Source: three-view drawing plus pictorial views. Frame: mm from the lowest corner of the part. Give positions to 0.01 mm unless a question says otherwise; leave off trailing zeros. Loops run counter-clockwise (first coordinate to the right, second up) from the corner with the lowest first, then second, coordinate; pieces in that order, holes last. Notation, with made-up numbers: (-37.75, 88.5) - (10.25, 88.5) arc R17 cw to (10.25, 98.5) - close; hole circle Ø2 at (77, -3). An arc over 180 degrees is marked (long way). Answer in a Markdown table with one row per item.
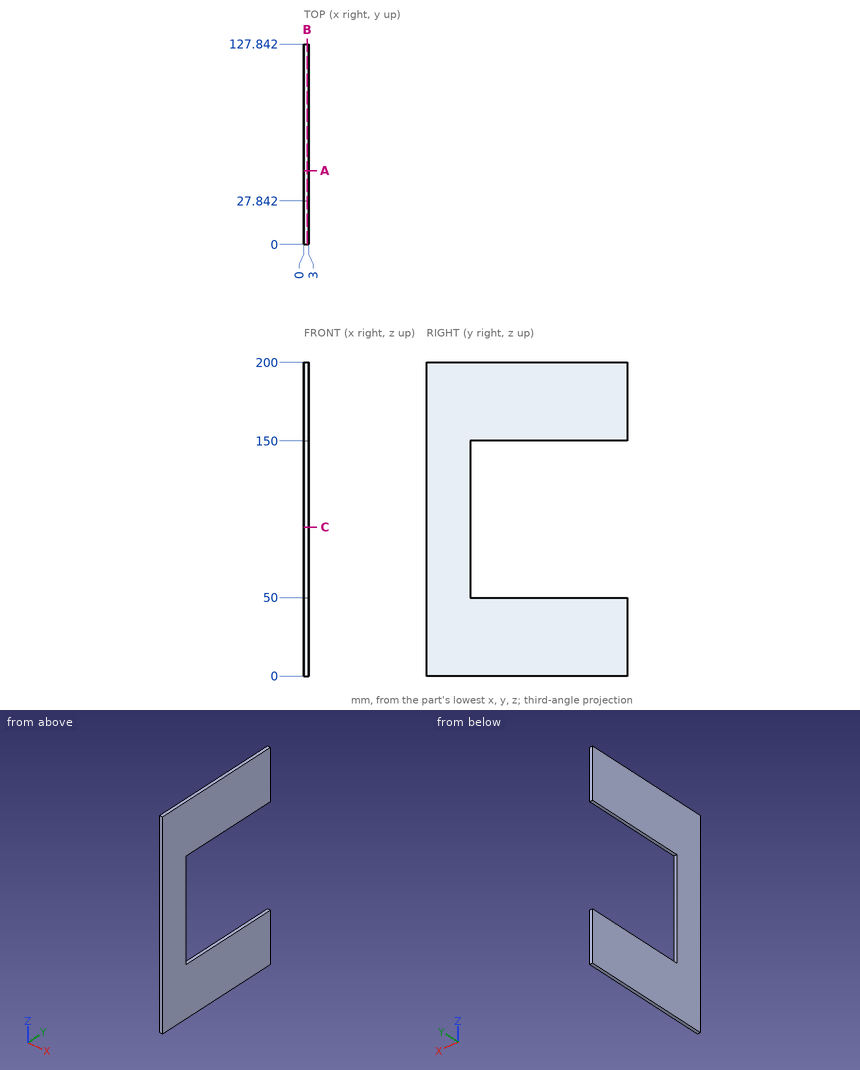
Q1. Material intervals for line 1 along Z through (x, y) = (1.8, 73.5); line 2 along Y through (x, z) = (1.45, 64.5), sorted ascending.
Check values:
| item | result |
|---|---|
| line 1 | 0 to 50, 150 to 200 |
| line 2 | 0 to 27.84 |
Q2. First-contact query: pin 1 (1.5 mm diameter, centred on x = 2, z = 76, fed in from +Y); pin 2 (1 mm diameter, centred on y = 13, z = 162.5, fed in from -X). Flat tips, straight axial feed; report the tip coordinate or a pass-through.
Check values:
| item | result |
|---|---|
| pin 1 | y = 27.84 |
| pin 2 | x = 0 |
Q3. Cut plane A-A (y = 47). Output: boundary loops of the cut face in (x, z), and give its area (3 significant figures).
Check values:
| item | result |
|---|---|
| outline | (0, 0) - (3, 0) - (3, 50) - (0, 50) - close; (0, 150) - (3, 150) - (3, 200) - (0, 200) - close |
| area | 300 mm² |
Q4. Cut plane B-B (x = 2.05). Output: boundary loops of the cut face in (y, z), and give its area (3 significant figures).
Check values:
| item | result |
|---|---|
| outline | (0, 0) - (127.84, 0) - (127.84, 50) - (27.84, 50) - (27.84, 150) - (127.84, 150) - (127.84, 200) - (0, 200) - close |
| area | 15,600 mm² |
Q5. Cut plane C-C (z = 95). Output: boundary loops of the cut face in (x, y), and give its area (3 significant figures).
Check values:
| item | result |
|---|---|
| outline | (0, 0) - (3, 0) - (3, 27.84) - (0, 27.84) - close |
| area | 83.5 mm² |
